Could you check a few things on this model? Use its own coordinates, in mm. A direction names the side the tool comes from. Round coordinates to 2 decimals unless told otherwise and drop trailing zeros. Loops run counter-clockwise (first coordinate to the right, second up) from the corner with the lowest first, then second, coordinate; pieces in that order, holes last. Notation, with made-up numbers: (68.25, 87) -> (83.25, 87) arc R24 ccw to (83.25, 108) -> close; hole circle Ø2 at (31.25, -21). An arc over 180 degrees is marked (long way). One line per item, written item: value.
```python
from build123d import *

# Parameters (mm, degrees)
BOSS_EXTRU_1_DEPTH      = 42.5
D_GAGEMENT_M31_D        = 3
ESQUISSE10_W            = 4
ESQUISSE10_H            = 10
BOSS_EXTRU_2_DEPTH      = 10
ESQUISSE12_R            = 6.075
ENL_V_MAT_EXTRU_3_DEPTH = 82.036925103
D_GAGEMENT_M33_D        = 3.4
ENL_V_MAT_EXTRU_1_DEPTH = 1.5
CHANFREIN1_SIZE         = 4
ESQUISSE13_W            = 8
ESQUISSE13_H            = 4
ENL_V_MAT_EXTRU_4_DEPTH = 81.362549025
ESQUISSE14_W            = 8.4
ESQUISSE14_H            = 14
BOSS_EXTRU_3_DEPTH      = 7.5
ESQUISSE15_R            = 4
ENL_V_MAT_EXTRU_5_DEPTH = 79.852350822
CONG_2_R                = 3
CONG_3_R                = 6
CONG_4_R                = 0.5
ESQUISSE16_W            = 4
ESQUISSE16_H            = 1.4
ENL_V_MAT_EXTRU_6_DEPTH = 67.151912076
CONG_5_R                = 3


# Some blends are built 0.0001 mm under size
with BuildPart() as part:
    # Esquisse1 → Boss.-Extru.1 (new body)
    with BuildSketch(Plane(origin=(0, 0, 0), x_dir=(1, 0, 0), z_dir=(0, 0, -1))):
        Polygon((-1.384510159, -46.220398701), (38.615489841, -46.220398701), (38.615489841, -42.220398701), (24.615489841, -42.220398701), (24.615489841, -36.220398701), (12.615489841, -36.220398701), (12.615489841, -42.220398701), (-1.384510159, -42.220398701), align=None)
    extrude(amount=BOSS_EXTRU_1_DEPTH)

    # Dégagement M31 (through all)
    with Locations(Plane(origin=(24.615489841, 0, 0), x_dir=(0, 0, -1), z_dir=(1, 0, 0))):
        with Locations((10, 39.220398701), (32.5, 39.220398701)):
            Hole(D_GAGEMENT_M31_D / 2)

    # Esquisse10 → Boss.-Extru.2 (add)
    with BuildSketch(Plane(origin=(0, 46.220398701, 0), x_dir=(1, 0, 0), z_dir=(0, 1, 0))):
        with Locations((32.215489841, 37.5)):
            Rectangle(ESQUISSE10_W, ESQUISSE10_H)
        Polygon((34.215489841, 10), (34.215489841, 0), (38.615489841, 0), (38.615489841, 42.5), (34.215489841, 42.5), (34.215489841, 32.5), align=None)
        with Locations((32.215489841, 5)):
            Rectangle(ESQUISSE10_W, ESQUISSE10_H)
    extrude(amount=BOSS_EXTRU_2_DEPTH)

    # Esquisse12 → Enlèv. mat.-Extru.3 (cut, through all)
    with BuildSketch(Plane(origin=(38.615489841, 0, 0), x_dir=(0, 0, -1), z_dir=(1, 0, 0))):
        with Locations((21.25, 56.220398701)):
            Circle(ESQUISSE12_R)
    extrude(amount=-ENL_V_MAT_EXTRU_3_DEPTH, mode=Mode.SUBTRACT)

    # Dégagement M33 (through all)
    with Locations(Plane(origin=(0, 42.220398701, 0), x_dir=(-1, 0, 0), z_dir=(0, -1, 0))):
        with Locations((3, -59.94627318), (-34.615489841, 38.5), (-2.615489841, 38.5), (-2.615489841, 4), (-34.615489841, 4)):
            Hole(D_GAGEMENT_M33_D / 2)

    # Esquisse9 → Enlèv. mat.-Extru.1 (cut)
    with BuildSketch(Plane.XZ.offset(-42.220398701)):
        Polygon((32.865489841, -35.468911087), (31.115489841, -38.5), (32.865489841, -41.531088913), (36.365489841, -41.531088913), (38.115489841, -38.5), (36.365489841, -35.468911087), align=None)
        Polygon((4.365489841, -35.468911087), (0.865489841, -35.468911087), (-0.884510159, -38.5), (0.865489841, -41.531088913), (4.365489841, -41.531088913), (6.115489841, -38.5), align=None)
        Polygon((32.865489841, -0.968911087), (31.115489841, -4), (32.865489841, -7.031088913), (36.365489841, -7.031088913), (38.115489841, -4), (36.365489841, -0.968911087), align=None)
        Polygon((4.365489841, -0.968911087), (0.865489841, -0.968911087), (-0.884510159, -4), (0.865489841, -7.031088913), (4.365489841, -7.031088913), (6.115489841, -4), align=None)
    extrude(amount=-ENL_V_MAT_EXTRU_1_DEPTH, mode=Mode.SUBTRACT)

    # Chanfrein1
    chanfrein1_edges = [part.edges().sort_by_distance(p)[0] for p in [
        (30.215489841, 51.220398701, -32.5),
        (30.215489841, 51.220398701, -10),
    ]]
    chamfer(chanfrein1_edges, length=CHANFREIN1_SIZE - 0.0001)  # a hair under: the kernel refuses the full size

    # Esquisse13 → Enlèv. mat.-Extru.4 (cut, through all)
    with BuildSketch(Plane(origin=(0, 0, -42.5), x_dir=(-1, 0, 0), z_dir=(0, 0, -1))):
        with Locations((-2.615489841, 44.220398701)):
            Rectangle(ESQUISSE13_W, ESQUISSE13_H)
    extrude(amount=-ENL_V_MAT_EXTRU_4_DEPTH, mode=Mode.SUBTRACT)

    # Esquisse14 → Boss.-Extru.3 (add)
    with BuildSketch(Plane(origin=(0, 0, -42.5), x_dir=(-1, 0, 0), z_dir=(0, 0, -1))):
        with Locations((-34.415489841, 49.220398701)):
            Rectangle(ESQUISSE14_W, ESQUISSE14_H)
    extrude(amount=BOSS_EXTRU_3_DEPTH)

    # Esquisse15 → Enlèv. mat.-Extru.5 (cut, through all)
    with BuildSketch(Plane.ZY.offset(-30.215489841)):
        with Locations((-46.7, 50.438462286)):
            Circle(ESQUISSE15_R)
    extrude(amount=-ENL_V_MAT_EXTRU_5_DEPTH, mode=Mode.SUBTRACT)

    # Congé2
    cong_2_edges = [part.edges().sort_by_distance(p)[0] for p in [
        (34.415489841, 56.220398701, -50),
    ]]
    fillet(cong_2_edges, radius=CONG_2_R)

    # Congé3
    # the kernel refuses this fillet: 6 mm, written as the material it takes off along each edge
    with BuildSketch(Plane(origin=(53.615489841, 42.220398701, -50), x_dir=(0, 1, 0), z_dir=(-1, 0, 0))) as cong_3_piece_1:
        with BuildLine():
            CenterArc((CONG_3_R, -CONG_3_R), CONG_3_R, 90, 90)
            Line((0, -CONG_3_R), (0, 0))
            Line((0, 0), (CONG_3_R, 0))
        make_face()
    extrude(amount=38.4, mode=Mode.SUBTRACT)

    # Congé4
    cong_4_edges = [part.edges().sort_by_distance(p)[0] for p in [
        (34.415489841, 52.698993197, -50),
        (34.415489841, 48.177709694, -49.999848135),
    ]]
    fillet(cong_4_edges, radius=CONG_4_R)

    # Esquisse16 → Enlèv. mat.-Extru.6 (cut, through all)
    with BuildSketch(Plane(origin=(0, 56.220398701, 0), x_dir=(1, 0, 0), z_dir=(0, 1, 0))):
        with Locations((34.415489841, 43.46034171)):
            Rectangle(ESQUISSE16_W, ESQUISSE16_H)
    extrude(amount=-ENL_V_MAT_EXTRU_6_DEPTH, mode=Mode.SUBTRACT)

    # Congé5
    cong_5_edges = [part.edges().sort_by_distance(p)[0] for p in [
        (30.215489841, 51.220398701, -36.4999),
        (30.215489841, 51.220398701, -6.0001),
    ]]
    fillet(cong_5_edges, radius=CONG_5_R)


solid = part.part
```
(1) Imagine slicing it at A-A on z = -28. Write out the boundary of the cut face in (x, y).
Results below:
outline: (6.62, 42.22) -> (12.62, 42.22) -> (12.62, 36.22) -> (24.62, 36.22) -> (24.62, 42.22) -> (38.62, 42.22) -> (38.62, 56.22) -> (34.22, 56.22) -> (34.22, 46.22) -> (6.62, 46.22) -> close
(2) On a 3-axis mill with a long thin cutter (end or side, diameter ignored), from which of +Z, -Z, +X, -X, +Y, -Y can I reach the whole of each face in a straight line? I mean faces 4 (the face through (34.215, 50, -21)), 5 (the face through (33, 43.72, -3)), 6 (the face through (36.415, 45, -43)). Say none if no direction works.
Results below:
face 4: -X, +Y
face 5: -Y
face 6: +Y, -Y
(3) Imagine slicing it at D-D on x = 28.5. Write out the boundary of the cut face in (y, z).
Results below:
outline: (42.22, -42.5) -> (46.22, -42.5) -> (46.22, 0) -> (42.22, 0) -> close
(4) We'd pull the mould along Y, two halves only. Please class faces 1 (the face through (18.53, 38.31, -11.19)), 2 (the face through (24.615, 39, -21)), 3 (the face through (34.47, 43.48, -47.68)): +Y half, -Y half, draft (parallel to the pull), parting line (faces both ways), or undercut.
Results below:
face 1: undercut
face 2: draft
face 3: -Y half
(5) For pin 1 Ø2 at (x, z) = (12.5, -10.5) entering from -Y; pin 2 Ø1.5 at (x, z) = (23.5, -29.5) entering from +Y; pin 3 Ø2.5 at (x, z) = (34.62, -4) entering from +Y; pin 4 Ø0.7 at (y, z) = (46, -43.5) entering from -X, each with a flat end and sliding along its axis, tell me the tip position at first contact or that it passes through.
Results below:
pin 1: stops at y = 36.22
pin 2: stops at y = 46.22
pin 3: passes through
pin 4: stops at x = 30.22
(6) Imagine slicing it at B-B on x = 21. Write out the boundary of the cut face in (y, z), then the cut area to 3 significant figures.
Results below:
outline: (36.22, -42.5) -> (46.22, -42.5) -> (46.22, 0) -> (36.22, 0) -> close; hole circle Ø3 at (39.22, -32.5); hole circle Ø3 at (39.22, -10)
area: 411 mm²
(7) Imagine slicing it at C-C on z = -21.25. Write out the boundary of the cut face in (x, y), then the cut area to 3 significant figures.
Results below:
outline: (6.62, 42.22) -> (12.62, 42.22) -> (12.62, 36.22) -> (24.62, 36.22) -> (24.62, 42.22) -> (38.62, 42.22) -> (38.62, 50.15) -> (34.22, 50.15) -> (34.22, 46.22) -> (6.62, 46.22) -> close
area: 217 mm²
(8) Please list where these lines run through material, in increasing order: L1, parallel to Y at x = 20, z = -10; L2, parallel to Z at x = 23.5, y = 40; L3, parallel to Y at x = 36, z = -8.
Results below:
L1: y = 36.22 to 37.72, 40.72 to 46.22
L2: z = -42.5 to -33.78, -31.22 to -11.28, -8.72 to 0
L3: y = 42.22 to 56.22
